Geometry check sheet. Reference: the model listing, model coordinates, mm. Face numbers are marked on the shaded views. A direction names the side the tool comes from. Coordinates: 2 decimals unless noted, no trailing zeros. Write each loop counter-clockwise with the first axis right and the second up, starting at its lowest first coordinate (ties: lowest second). Pieces come first, ordered by that corner, then holes. Notation, with made-up numbers: (-36.75, 34.25) -> (14.25, 34.25) arc R13 cw to (14.25, 44.25) -> close; hole circle Ø6 at (11, -32.5). An arc over 180 degrees is marked (long way). Put each result on its own line as item: value. Start each with the question number.
from build123d import *

# Parameters (mm, degrees)
F3_DEPTH = 50.8
F1_W     = 27.572012
F1_H     = 25.4
F4_DEPTH = 25.4
F2_W     = 25.4
F2_H     = 12.7
F5_DEPTH = 12.7


with BuildPart() as f3:
    # F0 (on Front) → F3 (new body)
    with BuildSketch(Plane.XZ):
        Polygon((0, 50.8), (0, 0), (76.2, 0), (76.2, 24.685946), (12.7, 24.685946), (12.7, 50.8), align=None)
    extrude(amount=-F3_DEPTH)

    # F1 (on Top) → F4 (cut)
    with BuildSketch(Plane.XY):
        with Locations((62.413994, 25.4)):
            Rectangle(F1_W, F1_H)
    extrude(amount=F4_DEPTH, mode=Mode.SUBTRACT)

    # F2 (on Right) → F5 (cut)
    with BuildSketch(Plane.YZ):
        with Locations((25.4, 44.45)):
            Rectangle(F2_W, F2_H)
    extrude(amount=F5_DEPTH, mode=Mode.SUBTRACT)


solid = f3.part
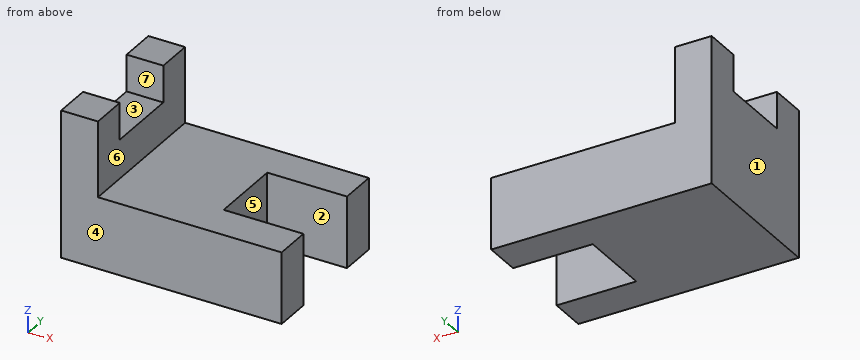
Item 1: Scan lines: line 1 along Y through (x, z) = (69, 19); line 2 along Z through (x, y) = (44, 45); line 3 along X through (y, z) = (42, 36). Record each from-to range of solid material in increasing order. Write a range as [from, to].
Item 2: Access from +Z, -Z, +X, -X, +Y, -Y to the whole of each face (thin tool, end or side, straight path). Record for the marked faces 5, 6 and 7.
Item 3: Mould release check, pull along Y, two halves, no side actions. Record for the marked faces 1, 2, 3 and 4: released by +Y, released by -Y, zero draft, split by the parting line, or undercut.
Item 4: Go/stop test with flat-tipped pins: P1, Ø6.5, axis at x = 9, y = 27.5, coming from the +Z side; P2, Ø7.5, axis at y = 19, z = 10.5, coming from the +X side; P3, Ø3, axis at y = 21.5, z = 41, coming from the -X side; P4, Ø13, axis at y = 35, z = 44, coming from the +X side. Record where each tip stops, or that it passes through.
Item 5: Section check B-B, the plane z = 41. Enter the section's corners in (x, y).
Item 6: Section check D-D, the plane y = 9. Enter the section's corners in (x, z), and give its area (3 significant figures).
Item 7: Section check C-C, the plane z = 6.5. Enter the section's corners in (x, y), and give its area (3 significant figures).
Item 8: Section check A-A, the plane x = 67.5. Enter the section's corners in (y, z), and give its area (3 significant figures).
From the geometry:
1. line 1: [0, 12.7], [38.1, 50.8]
1. line 2: [0, 24.69]
1. line 3: [0, 12.7]
2. face 5: +Z, -Z, +X
2. face 6: +Z, +X, +Y, -Y
2. face 7: +Z, +X, -X
3. face 1: zero draft
3. face 2: undercut
3. face 3: undercut
3. face 4: released by -Y
4. P1: z = 38.1
4. P2: x = 48.63
4. P3: through
4. P4: x = 12.7
5. outline: (0, 0) -> (12.7, 0) -> (12.7, 12.7) -> (0, 12.7) -> close; (0, 38.1) -> (12.7, 38.1) -> (12.7, 50.8) -> (0, 50.8) -> close
6. outline: (0, 0) -> (76.2, 0) -> (76.2, 24.69) -> (12.7, 24.69) -> (12.7, 50.8) -> (0, 50.8) -> close
6. area: 2,210 mm²
7. outline: (0, 0) -> (76.2, 0) -> (76.2, 12.7) -> (48.63, 12.7) -> (48.63, 38.1) -> (76.2, 38.1) -> (76.2, 50.8) -> (0, 50.8) -> close
7. area: 3,170 mm²
8. outline: (0, 0) -> (12.7, 0) -> (12.7, 24.69) -> (0, 24.69) -> close; (38.1, 0) -> (50.8, 0) -> (50.8, 24.69) -> (38.1, 24.69) -> close
8. area: 627 mm²
